Here's how the part is built. I have some questions about the finished solid (model axes, mm). Face numbers are marked on the shaded views. A direction names the side the tool comes from. Round coordinates to 2 decimals unless told otherwise and drop trailing zeros. Loops run counter-clockwise (first coordinate to the right, second up) from the corner with the lowest first, then second, coordinate; pieces in that order, holes last. Notation, with made-up numbers: (-16.5, -27.75) -> (32.5, -27.75) arc R18 cw to (32.5, -22.75) -> close; hole circle Ø11 at (23.5, -18). An arc over 180 degrees is marked (long way). One line per item, written item: value. Start each with the question number.
```python
from build123d import *

# Parameters (mm, degrees)
F1_DEPTH      = 31.75
F1_DEPTH_BACK = 31.75
F2_DEPTH      = 25.4
F2_DEPTH_BACK = 25.4
F3_R          = 6.35
F4_DEPTH      = 15.875
F5_R          = 6.35
F6_DEPTH      = 15.875
F7_W          = 186.001042
F7_H          = 50.8
F7_W_2        = 67.998958
F8_DEPTH      = 44.45


with BuildPart() as f1:
    # F0 (on Front) → F1 (new body, two sides)
    with BuildSketch(Plane.XZ) as f1_sk:
        with BuildLine():
            Line((0, -11.055585), (0, -6.35))
            ThreePointArc((0, -6.35), (4.490128, 4.490128), (-6.35, 0))
            Line((-6.35, 0), (-23.488146, 0))
            ThreePointArc((-23.488146, 0), (-25.145368, -0.220064), (-26.687727, -0.865004))
            Line((-26.687727, -0.865004), (-76.2, -29.747163))
            Line((-76.2, -29.747163), (-82.599162, -31.75))
            Line((-82.599162, -31.75), (-120.65, -31.75))
            ThreePointArc((-120.65, -31.75), (-123.825, -32.600739), (-126.149261, -34.925))
            ThreePointArc((-126.149261, -34.925), (-128.473523, -37.249261), (-131.648523, -38.1))
            Line((-131.648523, -38.1), (-152.4, -38.1))
            Line((-152.4, -38.1), (-355.6, -38.1))
            Line((-355.6, -38.1), (-374.65, -38.1))
            ThreePointArc((-374.65, -38.1), (-379.140128, -39.959872), (-381, -44.45))
            ThreePointArc((-381, -44.45), (-379.140128, -48.940128), (-374.65, -50.8))
            Line((-374.65, -50.8), (-131.648523, -50.8))
            ThreePointArc((-131.648523, -50.8), (-128.473523, -51.650739), (-126.149261, -53.975))
            ThreePointArc((-126.149261, -53.975), (-123.825, -56.299261), (-120.65, -57.15))
            Line((-120.65, -57.15), (-76.2, -57.15))
            Line((-76.2, -57.15), (-69.800838, -55.419992))
            Line((-69.800838, -55.419992), (-3.150419, -16.540581))
            ThreePointArc((-3.150419, -16.540581), (-0.843647, -14.218271), (0, -11.055585))
        make_face()
        with BuildLine():
            ThreePointArc((-4.7625, 0), (0, 4.7625), (4.7625, 0))
            ThreePointArc((4.7625, 0), (0, -4.7625), (-4.7625, 0))
        make_face(mode=Mode.SUBTRACT)
    extrude(amount=F1_DEPTH)
    extrude(f1_sk.sketch, amount=-F1_DEPTH_BACK)

    # F0 (on Front) → F2 (join, two sides)
    with BuildSketch(Plane.XZ) as f2_sk:
        with BuildLine():
            ThreePointArc((-4.7625, 0), (0, -4.7625), (4.7625, 0))
            ThreePointArc((4.7625, 0), (0, 4.7625), (-4.7625, 0))
        make_face()
        with BuildLine():
            Line((0, -11.055585), (0, -6.35))
            ThreePointArc((0, -6.35), (4.490128, 4.490128), (-6.35, 0))
            Line((-6.35, 0), (-23.488146, 0))
            ThreePointArc((-23.488146, 0), (-25.145368, -0.220064), (-26.687727, -0.865004))
            Line((-26.687727, -0.865004), (-76.2, -29.747163))
            Line((-76.2, -29.747163), (-82.599162, -31.75))
            Line((-82.599162, -31.75), (-120.65, -31.75))
            ThreePointArc((-120.65, -31.75), (-123.825, -32.600739), (-126.149261, -34.925))
            ThreePointArc((-126.149261, -34.925), (-128.473523, -37.249261), (-131.648523, -38.1))
            Line((-131.648523, -38.1), (-152.4, -38.1))
            Line((-152.4, -38.1), (-355.6, -38.1))
            Line((-355.6, -38.1), (-374.65, -38.1))
            ThreePointArc((-374.65, -38.1), (-379.140128, -39.959872), (-381, -44.45))
            ThreePointArc((-381, -44.45), (-379.140128, -48.940128), (-374.65, -50.8))
            Line((-374.65, -50.8), (-131.648523, -50.8))
            ThreePointArc((-131.648523, -50.8), (-128.473523, -51.650739), (-126.149261, -53.975))
            ThreePointArc((-126.149261, -53.975), (-123.825, -56.299261), (-120.65, -57.15))
            Line((-120.65, -57.15), (-76.2, -57.15))
            Line((-76.2, -57.15), (-69.800838, -55.419992))
            Line((-69.800838, -55.419992), (-3.150419, -16.540581))
            ThreePointArc((-3.150419, -16.540581), (-0.843647, -14.218271), (0, -11.055585))
        make_face()
        with BuildLine():
            ThreePointArc((-4.7625, 0), (0, 4.7625), (4.7625, 0))
            ThreePointArc((4.7625, 0), (0, -4.7625), (-4.7625, 0))
        make_face(mode=Mode.SUBTRACT)
        with BuildLine():
            Line((-355.6, -38.1), (-152.4, -38.1))
            Line((-152.4, -38.1), (-152.4, 0))
            Line((-152.4, 0), (-220.398958, 0))
            ThreePointArc((-220.398958, 0), (-226.142749, -1.926679), (-229.562879, -6.927273))
            ThreePointArc((-229.562879, -6.927273), (-254, -25.4), (-278.437121, -6.927273))
            ThreePointArc((-278.437121, -6.927273), (-281.857251, -1.926679), (-287.601042, 0))
            Line((-287.601042, 0), (-355.6, 0))
            Line((-355.6, 0), (-355.6, -38.1))
        make_face()
    extrude(amount=F2_DEPTH)
    extrude(f2_sk.sketch, amount=-F2_DEPTH_BACK)

    # F3 (on face) → F4 (cut)
    with BuildSketch(Plane(origin=(0, 31.75, 0), x_dir=(-1, 0, 0), z_dir=(0, 1, 0))):
        Circle(F3_R)
    extrude(amount=-F4_DEPTH, mode=Mode.SUBTRACT)

    # F5 (on face) → F6 (cut)
    with BuildSketch(Plane.XZ.offset(31.75)):
        Circle(F5_R)
    extrude(amount=-F6_DEPTH, mode=Mode.SUBTRACT)

    # F7 (on face) → F8 (cut)
    with BuildSketch(Plane.XY):
        with Locations((-313.399479, 0)):
            Rectangle(F7_W, F7_H)
        with Locations((-186.399479, 0)):
            Rectangle(F7_W_2, F7_H)
    extrude(amount=-F8_DEPTH, mode=Mode.SUBTRACT)


solid = f1.part
```
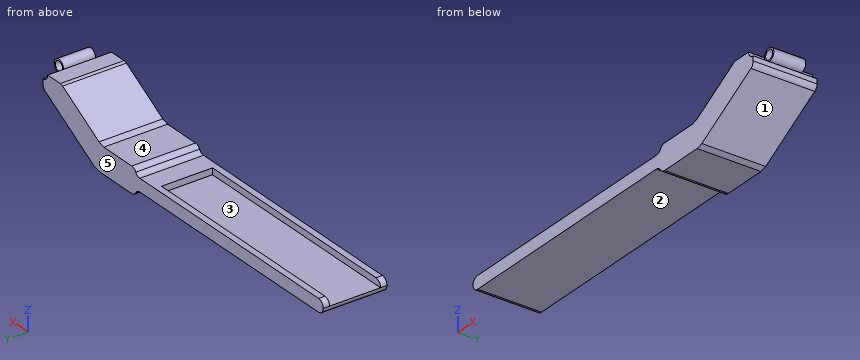
Q1. Which directions (+Z, -Z, +X, -X, +Y, -Y) give clear straight access to the entire face, cutting with the end or side of a thin tool? Please do the marked faces 1 and 2.
Q2. If we mould it in two halves opening along Y, with no side actions, what happens to the marked faces 3, 4 and 5? For each: released by +Y, released by -Y, zero draft, split by the parting line, or undercut.
Q3. If I drill on line 1 along Z through (x, y) = (-357, -15); line 2 along Y through (x, z) = (-341.5, -39); line 3 along Z through (x, y) = (-115, 23), over which ranges is the centre line in solid material (lowest first)?
Q4. Will these pins go through, and if not, where does the flat tip stop? P1, Ø3, axis at y = -4, z = -40, coming from the -X side; P2, Ø5, axis at y = 1, z = -8, coming from the -X side; P3, Ø6, axis at x = -321, y = -4.5, coming from the -Z side.
Q5. I want a section at D-D on z = -20.5. Please give me the cut outline in (x, y), plus the area to 3 significant figures.
Q6. I want a section at B-B on x = -300.5. Please give me the cut outline in (y, z).
Q7. I want a section at C-C on y = -22. Please give me the cut outline in (x, z) (3 decimals).
Answers below:
1. face 1: -Z, +X, +Y, -Y
1. face 2: -Z, -X, +Y, -Y
2. face 3: undercut
2. face 4: zero draft
2. face 5: released by +Y
3. line 1: z = -50.8 to -44.45
3. line 2: y = -31.75 to -25.4, 25.4 to 31.75
3. line 3: z = -57.15 to -31.75
4. P1: stops at x = -152.4
4. P2: stops at x = -43.2
4. P3: stops at z = -50.8
5. outline: (-60.35, -31.75) -> (-9.94, -31.75) -> (-9.94, 31.75) -> (-60.35, 31.75) -> close
5. area: 3,200 mm^2
6. outline: (-31.75, -50.8) -> (31.75, -50.8) -> (31.75, -38.1) -> (25.4, -38.1) -> (25.4, -44.45) -> (-25.4, -44.45) -> (-25.4, -38.1) -> (-31.75, -38.1) -> close
7. outline: (-381, -44.45) arc R6.35 ccw to (-374.65, -50.8) -> (-131.649, -50.8) arc R6.35 cw to (-126.149, -53.975) arc R6.35 ccw to (-120.65, -57.15) -> (-76.2, -57.15) -> (-69.801, -55.42) -> (-3.15, -16.541) arc R6.35 ccw to (0, -11.056) -> (0, -6.35) arc R6.35 cw to (-6.35, 0) -> (-23.488, 0) arc R6.35 ccw to (-26.688, -0.865) -> (-76.2, -29.747) -> (-82.599, -31.75) -> (-120.65, -31.75) arc R6.35 ccw to (-126.149, -34.925) arc R6.35 cw to (-131.649, -38.1) -> (-152.4, -38.1) -> (-152.4, -44.45) -> close
